Geometry: final body of the model. Coordinates: model frame, mm. A direction names the side the tool comes from. Round coordinates to 2 decimals unless told otherwise and drop trailing zeros. Write each loop counter-clockwise with the first axis right and the second up, starting at its lowest first coordinate (ties: lowest second). Pieces come first, ordered by that corner, then holes. Notation, with made-up numbers: M 12.5,84.25 L 30.5,84.25 A16 cw 30.5,92.25 Z; hole C 13.5,72.25 d3. An arc over 180 degrees is marked long. Use one line per item in the form item = value. Start each with the question number.
Item 1: Pin query (flat end, axial travel): pin 1 Ø5.5 at (x, y) = (-342.9, 149.225) entering from +Z (3 decimals); pin 2 Ø6.5 at (x, z) = (-98.425, 28.575) entering from -Y (3 decimals). Return the tip coordinate at first contact, or that it passes through.
Item 2: Section query A-A (x = 76). Return loops of the section in (y, z) (3 decimals).
Item 3: Reachability of faces 1 (the cylindrical face through (5.33, 175.25, 2.26)), 2 (the flat face through (-5, -4, 3.175)) from +Z, -Z, +X, -X, +Y, -Y: full face, straight path, thin tool, end or side. Return the list, or none.
Item 4: Section query C-C (y = -75). Return loops of the section in (x, z) (3 decimals), and give its area (3 significant figures).
Item 5: Section query B-B (z = 152.5). Return loops of the section in (x, y) (3 decimals), and give its area (3 significant figures).
Item 6: Ray query, probe 1 along Y at (x, z) = (-4, 345) (3 decimals); probe 2 along Z at (x, y) = (139, 42) (3 decimals); probe 3 along Y at (x, z) = (-342, 1) (3 decimals). Return the intervals inside material, ascending.
from build123d import *

# Parameters (mm, degrees)
SKETCH1_W                        = 762
SKETCH1_H                        = 349.25
BOSS_EXTRUDE1_DEPTH              = 3.175
EDGE_FLANGE1_STRIP_W             = 50.8
EDGE_FLANGE1_STRIP_H             = 6.35
EDGE_FLANGE1_STRIP_CUT_DEPTH     = 762
EDGE_FLANGE1_DEPTH               = 762
F_27_64_0_42188_DIAMETER_HOLE1_D = 10.715752
F_10_0_1935_DIAMETER_HOLE1_D     = 4.9149
F_10_0_1935_DIAMETER_HOLE2_D     = 4.9149
FILLET1_R                        = 6.35


# Sheet-metal steps are written as plain solids
with BuildPart() as part:
    # Sketch1 → Boss-Extrude1 (new, symmetric)
    with BuildSketch(Plane.XY):
        Rectangle(SKETCH1_W, SKETCH1_H)
    extrude(amount=BOSS_EXTRUDE1_DEPTH, both=True)

    # Edge-Flange1 strip (across the edge) → Edge-Flange1 strip cut (cut)
    with BuildSketch(Plane(origin=(381, 174.625, 3.175), x_dir=(0, -1, 0), z_dir=(-1, 0, 0))):
        with Locations((-12.7, -3.175)):
            Rectangle(EDGE_FLANGE1_STRIP_W, EDGE_FLANGE1_STRIP_H)
    extrude(amount=EDGE_FLANGE1_STRIP_CUT_DEPTH, mode=Mode.SUBTRACT)

    # Edge-Flange1 section (across the edge) → Edge-Flange1 (add)
    with BuildSketch(Plane(origin=(381, 174.625, 3.175), x_dir=(0, -1, 0), z_dir=(-1, 0, 0))):
        with BuildLine():
            Line((-6.35, 12.7), (-6.35, 482.6))
            Line((-6.35, 482.6), (0, 482.6))
            Line((0, 482.6), (0, 12.7))
            ThreePointArc((0, 12.7), (3.719743879, 3.719743879), (12.7, 0))
            Line((12.7, 0), (12.7, -6.35))
            ThreePointArc((12.7, -6.35), (-0.770384182, -0.770384182), (-6.35, 12.7))
        make_face()
    extrude(amount=EDGE_FLANGE1_DEPTH)

    # 27/64 (0.42188) Diameter Hole1 (through all)
    with Locations(Plane(origin=(0, 0, -3.175), x_dir=(-1, 0, 0), z_dir=(0, 0, -1))):
        with Locations((-31.75, -155.575), (336.55, -155.575), (31.75, -155.575), (-336.55, -155.575)):
            Hole(F_27_64_0_42188_DIAMETER_HOLE1_D / 2)

    # #10 (0.1935) Diameter Hole1 (through all)
    with Locations(Plane(origin=(0, 0, -3.175), x_dir=(-1, 0, 0), z_dir=(0, 0, -1))):
        with Locations((-342.9, 149.225), (-114.3, 149.225), (114.3, 149.225), (342.9, 149.225)):
            Hole(F_10_0_1935_DIAMETER_HOLE1_D / 2)

    # #10 (0.1935) Diameter Hole2 (through all)
    with Locations(Plane(origin=(0, 180.975, 0), x_dir=(1, 0, 0), z_dir=(0, 1, 0))):
        with Locations((-339.725, -28.575), (-98.425, -28.575), (98.425, -28.575), (339.725, -28.575)):
            Hole(F_10_0_1935_DIAMETER_HOLE2_D / 2)

    # Fillet1
    fillet1_edges = [part.edges().sort_by_distance(p)[0] for p in [
        (381, 177.8, 485.775),
        (-381, 177.8, 485.775),
        (381, -174.625, 0),
        (-381, -174.625, 0),
    ]]
    fillet(fillet1_edges, radius=FILLET1_R)


solid = part.part
Working result:
q1.pin_1 = 3.175
q1.pin_2 = 174.625
q2.outline = M -174.625,-3.175 L 161.925,-3.175 A19.05 ccw 180.975,15.875 L 180.975,485.775 L 174.625,485.775 L 174.625,15.875 A12.7 cw 161.925,3.175 L -174.625,3.175 Z
q3.face_1 = -Z, +X, -X, +Y
q3.face_2 = +Z, +X, -X, -Y
q4.outline = M -381,-3.175 L 381,-3.175 L 381,3.175 L -381,3.175 Z
q4.area = 4,840 mm²
q5.outline = M -381,174.625 L 381,174.625 L 381,180.975 L -381,180.975 Z
q5.area = 4,840 mm²
q6.probe_1 = 174.625 to 180.975
q6.probe_2 = -3.175 to 3.175
q6.probe_3 = -174.625 to 146.938, 151.512 to 173.826
